from build123d import *

# Parameters (mm, degrees)
SKETCH021_R     = 2.55
PAD_DEPTH       = 17
SKETCH022_R     = 2.55
SKETCH022_R_2   = 20.5
PAD004_DEPTH    = 2.5
POCKET006_DEPTH = 3
SKETCH024_R     = 2.2
POCKET007_DEPTH = 13.001
SKETCH025_R     = 3.2
POCKET008_DEPTH = 4
SKETCH026_R     = 4
POCKET009_DEPTH = 4
SKETCH027_R     = 4
POCKET010_DEPTH = 2
PAD007_DEPTH    = 4.9
CHAMFER005_SIZE = 0.5
CHAMFER006_SIZE = 0.3


with BuildPart() as part:
    # Sketch021 → Pad (new body)
    with BuildSketch(Plane.XY.offset(11.5)):
        with BuildLine():
            ThreePointArc((30, 43.542487), (0, 110), (-30, 43.542487))
            Line((-30, 43.542487), (-30, 26.457513))
            ThreePointArc((-30, 26.457513), (0, -40), (30, 26.457513))
            Line((30, 26.457513), (30, 43.542487))
        make_face()
        with BuildLine():
            ThreePointArc((20.001597, 37.69), (0, 108), (-20.001597, 37.69))
            Line((-20.001597, 37.69), (-20.001597, 32.31))
            ThreePointArc((-20.001597, 32.31), (0, -38), (20.001597, 32.31))
            Line((20.001597, 32.31), (20.001597, 37.69))
        make_face(mode=Mode.SUBTRACT)
        with Locations((-25, 35)):
            Circle(SKETCH021_R, mode=Mode.SUBTRACT)
        with Locations((25, 35)):
            Circle(SKETCH021_R, mode=Mode.SUBTRACT)
    extrude(amount=PAD_DEPTH)

    # Sketch022 → Pad004 (join)
    with BuildSketch(Plane.XY.offset(27.5)):
        with BuildLine():
            ThreePointArc((30, 43.542487), (0, 110), (-30, 43.542487))
            Line((-30, 43.542487), (-30, 26.457513))
            ThreePointArc((-30, 26.457513), (0, -40), (30, 26.457513))
            Line((30, 43.542487), (30, 26.457513))
        make_face()
        with Locations((-25, 35)):
            Circle(SKETCH022_R, mode=Mode.SUBTRACT)
        with Locations((25, 35)):
            Circle(SKETCH022_R, mode=Mode.SUBTRACT)
        with Locations((0, 70)):
            Circle(SKETCH022_R_2, mode=Mode.SUBTRACT)
    extrude(amount=PAD004_DEPTH)

    # Sketch020 → Revolution005 (revolve)
    with BuildSketch(Plane.YZ):
        Polygon((12.5, 23.25), (13.073063, 20), (28.677548, 20), (30, 27.5), (11.05, 27.5), (11.05, 24.9), (2.8, 24.9), (2.8, 15.9), (3.45, 15.9), (3.95, 16.4), (3.95, 23), (5.5, 23), (5.5, 23.25), align=None)
    revolve(axis=Axis((0, 0, 0), (0, 0, 1)))

    # Sketch023 → Pocket006 (cut)
    with BuildSketch(Plane.XY.offset(30)):
        with BuildLine():
            ThreePointArc((16.655, -21.25), (19.091248, -19.091248), (21.25, -16.655))
            Line((21.25, 16.655), (21.25, -16.655))
            ThreePointArc((21.25, 16.655), (19.091248, 19.091248), (16.655, 21.25))
            Line((-16.655, 21.25), (16.655, 21.25))
            ThreePointArc((-16.655, 21.25), (-19.091248, 19.091248), (-21.25, 16.655))
            Line((-21.25, -16.655), (-21.25, 16.655))
            ThreePointArc((-21.25, -16.655), (-19.091248, -19.091248), (-16.655, -21.25))
            Line((16.655, -21.25), (-16.655, -21.25))
        make_face()
    extrude(amount=-POCKET006_DEPTH, mode=Mode.SUBTRACT)

    # Sketch024 → Pocket007 (cut, through all)
    with BuildSketch(Plane.XY.offset(17)):
        with Locations((15.5, 15.5)):
            Circle(SKETCH024_R)
        with Locations((15.5, -15.5)):
            Circle(SKETCH024_R)
        with Locations((-15.5, -15.5)):
            Circle(SKETCH024_R)
        with Locations((-15.5, 15.5)):
            Circle(SKETCH024_R)
    extrude(amount=POCKET007_DEPTH, mode=Mode.SUBTRACT)

    # Sketch025 → Pocket008 (cut)
    with BuildSketch(Plane.XY.offset(20)):
        with Locations((15.5, 15.5)):
            Circle(SKETCH025_R)
        with Locations((15.5, -15.5)):
            Circle(SKETCH025_R)
        with Locations((-15.5, -15.5)):
            Circle(SKETCH025_R)
        with Locations((-15.5, 15.5)):
            Circle(SKETCH025_R)
    extrude(amount=POCKET008_DEPTH, mode=Mode.SUBTRACT)

    # Sketch026 (on Face12 of Pocket008) → Pocket009 (cut)
    with BuildSketch(Plane.XY.offset(30)):
        with Locations((25, 35)):
            Circle(SKETCH026_R)
        with Locations((-25, 35)):
            Circle(SKETCH026_R)
    extrude(amount=-POCKET009_DEPTH, mode=Mode.SUBTRACT)

    # Sketch027 (on Face1 of Pocket009) → Pocket010 (cut)
    with BuildSketch(Plane(origin=(0, 0, 11.5), x_dir=(1, 0, 0), z_dir=(0, 0, -1))):
        with Locations((-25, -35)):
            Circle(SKETCH027_R)
        with Locations((25, -35)):
            Circle(SKETCH027_R)
    extrude(amount=-POCKET010_DEPTH, mode=Mode.SUBTRACT)

    # Sketch032 → Pad007 (join)
    with BuildSketch(Plane(origin=(0, 70, 11.5), x_dir=(1, 0, 0), z_dir=(0, 0, 1))):
        with BuildLine():
            ThreePointArc((27.15203, -29.3729), (0, 40), (-27.15203, -29.3729))
            Line((-25.794428, -27.904255), (-27.15203, -29.3729))
            ThreePointArc((25.794428, -27.904255), (0, 38), (-25.794428, -27.904255))
            Line((25.794428, -27.904255), (27.15203, -29.3729))
        make_face()
        with BuildLine():
            ThreePointArc((-27.15203, -40.6271), (0, -110), (27.15203, -40.6271))
            Line((27.15203, -40.6271), (25.794428, -42.095745))
            ThreePointArc((-25.794428, -42.095745), (0, -108), (25.794428, -42.095745))
            Line((-27.15203, -40.6271), (-25.794428, -42.095745))
        make_face()
    extrude(amount=-PAD007_DEPTH)

    # Chamfer005
    chamfer005_edges = [part.edges().sort_by_distance(p)[0] for p in [
        (-30, 35, 30),
        (0, -40, 30),
        (0, 110, 30),
        (30, 35, 30),
        (0, 21.25, 30),
        (-19.091248, 19.091248, 30),
        (-21.25, 0, 30),
        (19.091248, -19.091248, 30),
        (21.25, 0, 30),
        (19.091248, 19.091248, 30),
        (-19.091248, -19.091248, 30),
        (0, -21.25, 30),
        (-20.5, 70, 30),
        (0, -11.05, 27),
        (0, -2.8, 24.9),
        (-20.5, 70, 27.5),
        (0, -38, 6.6),
        (0, 108, 6.6),
        (0, -13.073063, 20),
        (0, 108, 27.5),
        (20.001597, 35, 27.5),
        (0, -38, 27.5),
        (-20.001597, 35, 27.5),
        (-18.7, 15.5, 20),
        (-18.7, -15.5, 20),
        (12.3, -15.5, 20),
        (12.3, 15.5, 20),
        (21, 35, 11.5),
        (-29, 35, 11.5),
    ]]
    chamfer(chamfer005_edges, length=CHAMFER005_SIZE)

    # Chamfer006
    chamfer006_edges = [part.edges().sort_by_distance(p)[0] for p in [
        (-29, 35, 30),
        (21, 35, 30),
        (-17.7, -15.5, 27),
        (13.3, -15.5, 27),
        (13.3, 15.5, 27),
        (-17.7, 15.5, 27),
    ]]
    chamfer(chamfer006_edges, length=CHAMFER006_SIZE)


with BuildPart() as part_1:
    # Body007 placement: moved
    add(part.part.moved(Location((0, -70, 0))))


solid = part_1.part
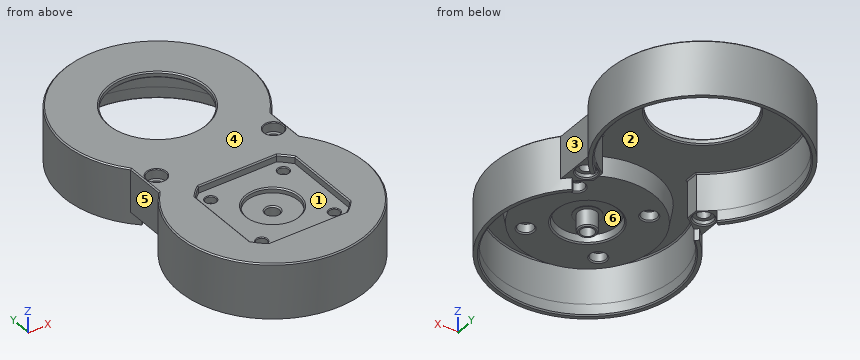
Design review of the part built by this model. Coordinates are the model's own, in mm. Face numbers are marked on the shaded views. A direction names the side the tool comes from. Give positions to 0.01 mm unless a question says otherwise; leave off trailing zeros. Order: outer loops, then holes, each group sorted by start corner. A loop starts at its lowest first (then second) coordinate and runs counter-clockwise, first axis right, second up.
1. Add section B-B, the plane y = -35. State how many separate pieces and enclosed holes the cut face has, then the cut area to 3 significant figures.
Solution:
separate pieces: 3
enclosed holes: 0
area: 246 mm2
2. For pin 1 Ø6 at (x, y) = (14.5, -66) entering from -Z; pin 2 Ø3 at (x, z) = (-6.5, 14) entering from -Y; pin 3 Ø10 at (y, z) = (-93.5, 10.5) entering from +X; pin 4 Ø3.5 at (x, y) = (0, -70) entering from -Z, all flat-tipped, find the tip position at first contact; note any pin that passes through.
Solution:
pin 1: stops at z = 20
pin 2: stops at y = -109.69
pin 3: stops at x = 35.46
pin 4: passes through
3. Add section A-A, the plane z = 18.25. State the section outline as (x, y) points, then the cut area to 3 significant figures.
Solution:
outline: (-30, -43.54) arc R40 ccw (long way) to (30, -43.54) - (30, -26.46) arc R40 ccw (long way) to (-30, -26.46) - close; circle Ø7.9 at (0, -70); hole circle Ø5.1 at (-25, -35); hole (-20, -37.69) arc R38 ccw (long way) to (20, -37.69) - (20, -32.31) arc R38 ccw (long way) to (-20, -32.31) - close; hole circle Ø5.6 at (0, -70); hole circle Ø5.1 at (25, -35)
area: 956 mm2
4. To check wall thickness, follow L1, parallel to X at y = -35, z = 18; L2, parallel to Y at x = -35, z = 26.5; L3, parallel to X at y = -59.5, z = 20.25. State the ranges of each line that lie inside material, in increasing order.
Solution:
L1: x = -30 to -27.55, -22.45 to -20, 20 to 22.45, 27.55 to 30
L2: y = -89.36 to -84.8, -55.2 to -50.64, -19.36 to -14.8, 14.8 to 19.36
L3: x = -38.6 to -36.52, -26.73 to -8.12, 8.12 to 26.73, 36.52 to 38.6
5. Mouldability with a two-part tool opening along X and no side actions: class the marked faces 3, 4, 5 and 6 as +X half, -X half, draft (parallel to the pull), parting line (faces both ways), or undercut.
Solution:
face 3: +X half
face 4: draft
face 5: -X half
face 6: undercut
6. Tool access review of the marked faces 1 and 2: name each direction out of +Z, -Z, +X, -X, +Y, -Y from which nothing blocks a thin tool from reaching the whole face with its end or side.
Solution:
face 1: +Z
face 2: -Z
